The listing builds one solid part. Answer for the finished solid, in the listing's coordinates (mm). Face numbers are marked on the shaded views. A direction names the side the tool comes from. Give positions to 0.01 mm unless a question says otherwise; leave off trailing zeros. Write each loop counter-clockwise with the first axis right and the second up, starting at its lowest first coordinate (ties: lowest second). Pieces come first, ordered by that corner, then holes. Notation, with made-up numbers: (37, 43) -> (86, 43) arc R24 ccw to (86, 67) -> close; hole circle Ø4 at (-14.5, 5.25). An arc over 180 degrees is marked (long way). Put each result on its own line as item: value. Start each with the question number.
1) A cutting plane is placed at A-A (y = 0). Write down the section's boundary in (x, z), then the cut area to 3 significant figures.
2) For the marked faces 1 and 2, determine the directions among +Z, -Z, +X, -X, +Y, -Y from which every point of the face is accessible in a straight line to the end or side of a thin tool.
3) Find the intervals of material crossed by line 1 along Z through (x, y) = (-1, 4.5); line 2 along Z through (x, y) = (6, 19); line 3 along Y through (x, z) = (1, -12), in increasing order. Write a range as from..to.
4) Flat-ended cylindrical pins translate along their axes: pin 1 Ø8 at (x, y) = (-5.5, -9) entering from -Z; pin 2 Ø8 at (y, z) = (0, -14) entering from +X; pin 3 Ø1.5 at (x, z) = (0, -14.5) entering from -Y. Find the tip coordinate at first contact, or state that the pin passes through.
5) A cutting plane is placed at C-C (z = -19.5). Write down the section's boundary in (x, y).
6) A cutting plane is placed at D-D (y = -12). Write down the section's boundary in (x, z), then the cut area to 3 significant figures.
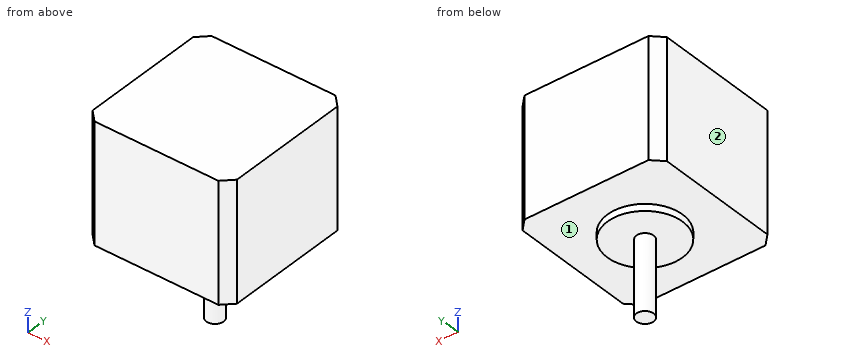
from build123d import *

# Parameters (mm, degrees)
F0_W     = 42.3
F0_H     = 42.3
F0_R     = 11
F0_R_2   = 2.5
F1_DEPTH = 35
F2_DEPTH = 24
F3_DEPTH = 2
F4_SIZE  = 3


with BuildPart() as f1:
    # F0 (on Top) → F1 (new body)
    with BuildSketch(Plane.XY):
        Rectangle(F0_W, F0_H)
        Circle(F0_R, mode=Mode.SUBTRACT)
        Circle(F0_R)
        Circle(F0_R_2, mode=Mode.SUBTRACT)
        Circle(F0_R_2)
    extrude(amount=F1_DEPTH)

    # F0 (on Top) → F2 (join)
    with BuildSketch(Plane.XY):
        Circle(F0_R_2)
    extrude(amount=-F2_DEPTH)

    # F0 (on Top) → F3 (join)
    with BuildSketch(Plane.XY):
        Circle(F0_R)
        Circle(F0_R_2, mode=Mode.SUBTRACT)
    extrude(amount=-F3_DEPTH)

    # F4
    f4_edges = [f1.edges().sort_by_distance(p)[0] for p in [
        (-21.15, -21.15, 17.5),
        (21.15, -21.15, 17.5),
        (21.15, 21.15, 17.5),
        (-21.15, 21.15, 17.5),
    ]]
    chamfer(f4_edges, length=F4_SIZE)


solid = f1.part
Reply:
1. outline: (-21.15, 0) -> (-11, 0) -> (-11, -2) -> (-2.5, -2) -> (-2.5, -24) -> (2.5, -24) -> (2.5, -2) -> (11, -2) -> (11, 0) -> (21.15, 0) -> (21.15, 35) -> (-21.15, 35) -> close
1. area: 1,630 mm2
2. face 1: -Z
2. face 2: +Z, -Z, -X, +Y, -Y
3. line 1: z = -2..35
3. line 2: z = 0..35
3. line 3: y = -2.29..2.29
4. pin 1: stops at z = -2
4. pin 2: stops at x = 2.5
4. pin 3: stops at y = -2.5
5. outline: circle Ø5 at (0, 0)
6. outline: (-21.15, 0) -> (21.15, 0) -> (21.15, 35) -> (-21.15, 35) -> close
6. area: 1,480 mm2
